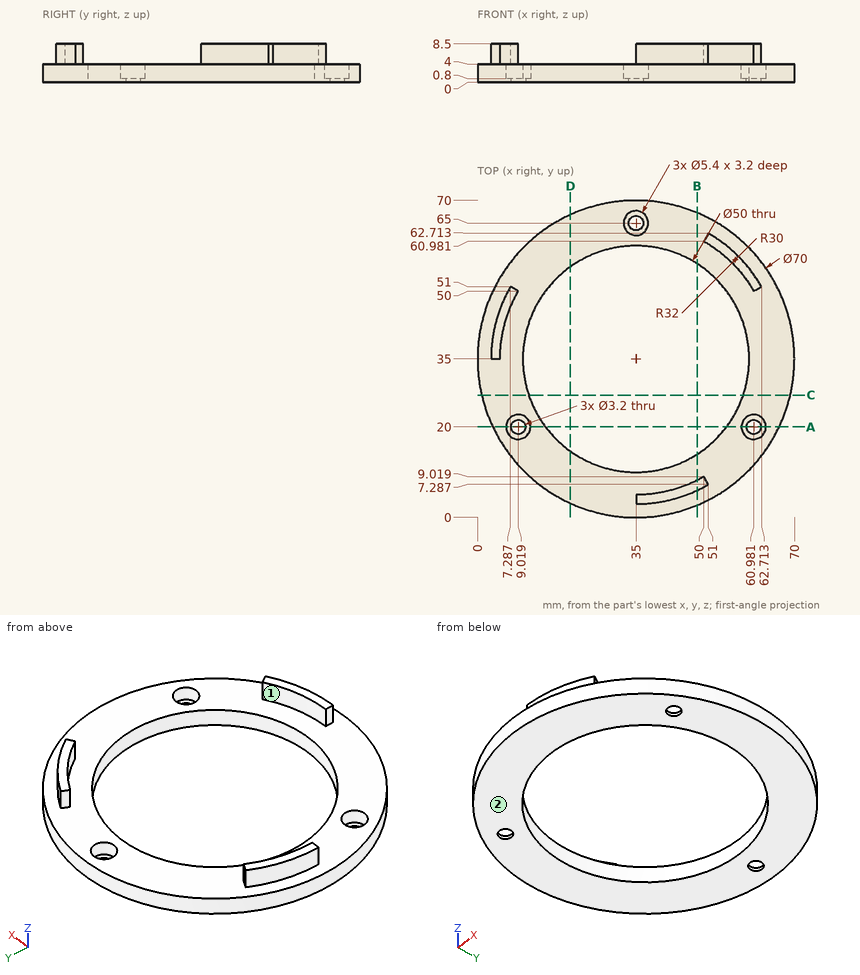
Can you work these out from the drawing? Everything is in mm from the part's minimum corner. Round coordinates to 2 decimals unless told otherwise and drop trailing zeros. Write each loop counter-clockwise with the first axis right and the second up, starting at its lowest first coordinate (ties: lowest second). Pieces come first, ordered by that corner, then holes.
1. Suppose I cut it at B-B (x = 48.5). List the corners of the cut face in (y, z) for me.
2. If we mould it in two halves opening along Y, with no side actions, what happens to the marked faces 1 and 2? For each: released by +Y, released by -Y, zero draft, split by the parting line, or undercut.
3. Will these pins go through, and if not, where does the flat tip stop? pin 1 Ø12 at (x, y) = (16, 48) entering from +Z; pin 2 Ø2 at (y, z) = (29, 4.5) entering from -X; pin 3 Ø2 at (x, z) = (3.5, 6.5) entering from -Y; pin 4 Ø2.5 at (x, y) = (35, 65) entering from -Z.
4. Suppose I cut it at A-A (y = 20). List the corners of the cut face in (x, z) for me.
5. Suppose I cut it at C-C (y = 27). List the corners of the cut face in (x, z) for me (1 decimal), and give its area (3 significant figures).
6. Suppose I cut it at D-D (x = 20.5). List the corners of the cut face in (y, z) for me (1 decimal).
7. I need wall thicknesses on L1, parallel to Y at x = 35, z = 3.05; L2, parallel to Y at x = 35, z = 0.6; L3, parallel to X at y = 22, z = 1 (1 decimal). Which ranges of each line are inside material? Lowest first, please.
Answer sheet:
1. outline: (2.71, 0) - (13.96, 0) - (13.96, 4) - (8.21, 4) - (8.21, 8.5) - (5.99, 8.5) - (5.99, 4) - (2.71, 4) - close; (56.04, 0) - (67.29, 0) - (67.29, 4) - (56.04, 4) - close
2. face 1: released by +Y
2. face 2: zero draft
3. pin 1: stops at z = 4
3. pin 2: stops at x = 0.38
3. pin 3: stops at y = 35
3. pin 4: passes through
4. outline: (3.38, 0) - (7.42, 0) - (7.42, 0.8) - (6.32, 0.8) - (6.32, 4) - (3.38, 4) - close; (10.62, 0) - (15, 0) - (15, 4) - (11.72, 4) - (11.72, 0.8) - (10.62, 0.8) - close; (55, 0) - (59.38, 0) - (59.38, 0.8) - (58.28, 0.8) - (58.28, 4) - (55, 4) - close; (62.58, 0) - (66.62, 0) - (66.62, 4) - (63.68, 4) - (63.68, 0.8) - (62.58, 0.8) - close
5. outline: (0.9, 0) - (11.3, 0) - (11.3, 4) - (0.9, 4) - close; (58.7, 0) - (69.1, 0) - (69.1, 4) - (58.7, 4) - close
5. area: 83.1 mm2
6. outline: (3.1, 0) - (14.6, 0) - (14.6, 4) - (3.1, 4) - close; (55.4, 0) - (66.9, 0) - (66.9, 4) - (55.4, 4) - close
7. L1: y = 0 to 10, 60 to 62.3, 67.7 to 70
7. L2: y = 0 to 10, 60 to 63.4, 66.6 to 70
7. L3: x = 2.5 to 7.2, 10.8 to 13.6, 56.4 to 59.2, 62.8 to 67.5
